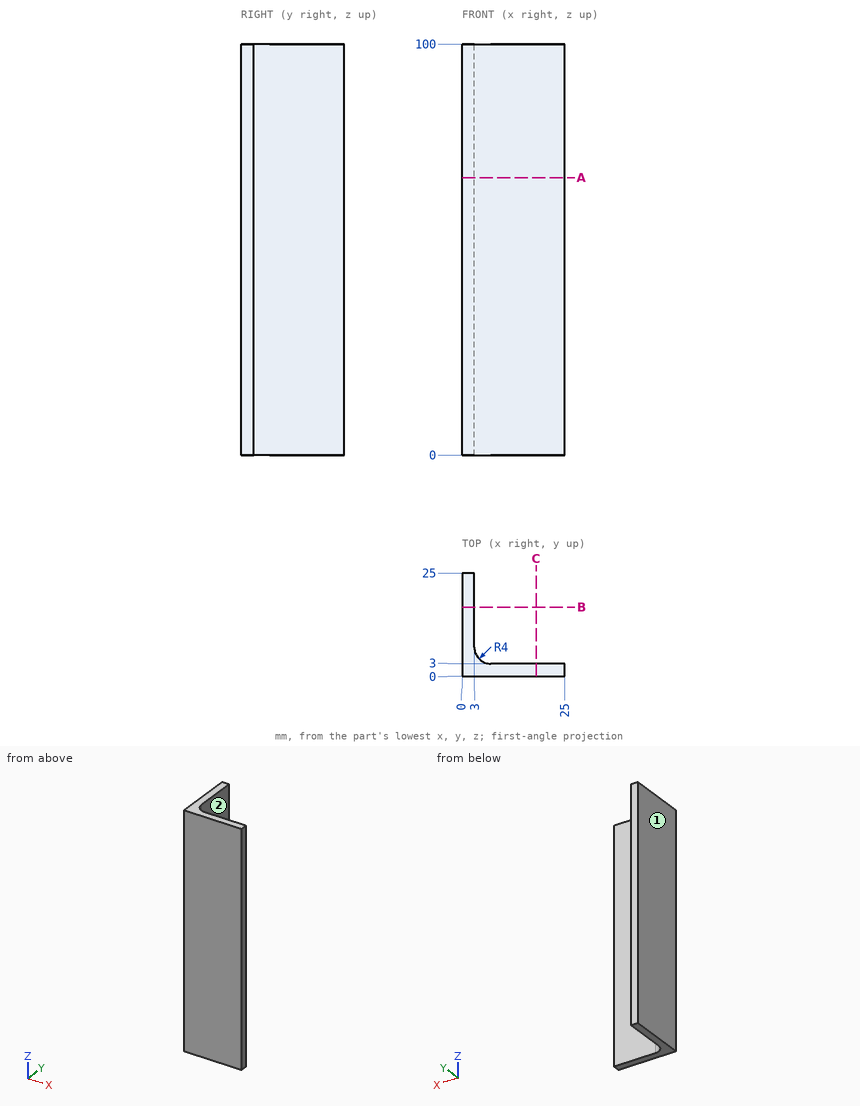
For this review, use the dimensioned drawing (mm, ordinates from the lowest corner) and the shaded views. A direction names the side the tool comes from. Round coordinates to 2 decimals unless told otherwise and drop trailing zeros. Write each loop counter-clockwise with the first axis right and the second up, starting at its lowest first coordinate (ties: lowest second). Pieces come first, ordered by that corner, then holes. Notation, with made-up numbers: M 47.5,76.25 L 100.5,76.25 A21 cw 100.5,111.25 Z; hole C 88,-2 d4. An arc over 180 degrees is marked long. Answer as CSV lines item,"result". Start each with the question number.
Q1. Tool access review of the marked faces 1 and 2: name each direction out of +Z, -Z, +X, -X, +Y, -Y from which nothing blocks a thin tool from reaching the whole face with its end or side.
Q2. Consider section B-B, the plane y = 16.75. Give the boundary of the cut face in (x, z), then the cut area to 3 significant figures.
Q3. Consider section A-A, the plane z = 67.5. Give the boundary of the cut face in (x, y), then the cut area to 3 significant figures.
Q4. Wall thickness on line 1 along X through (y, z) = (21, 67.5); line 2 along X through (y, z) = (5.25, 46): over which ranges is each line inside the solid? List them lowest first.
Q5. Clearance check with flat-ended pins moving along their axes: P1, Ø9, axis at y = 13.5, z = 55.5, coming from the +X side; P2, Ø5, axis at x = 9.5, z = 61, coming from the +Y side. State where each tip first meets the part, or that it passes through.
Result set:
1,face 1,"+Z, -Z, -X, +Y, -Y"
1,face 2,"+Z, -Z, +X, +Y"
2,outline,"M 0,0 L 3,0 L 3,100 L 0,100 Z"
2,area,"300 mm²"
3,outline,"M 0,0 L 25,0 L 25,3 L 7,3 A4 cw 3,7 L 3,25 L 0,25 Z"
3,area,"144 mm²"
4,line 1,"x = 0 to 3"
4,line 2,"x = 0 to 3.4"
5,P1,"stops at x = 3"
5,P2,"stops at y = 3"
